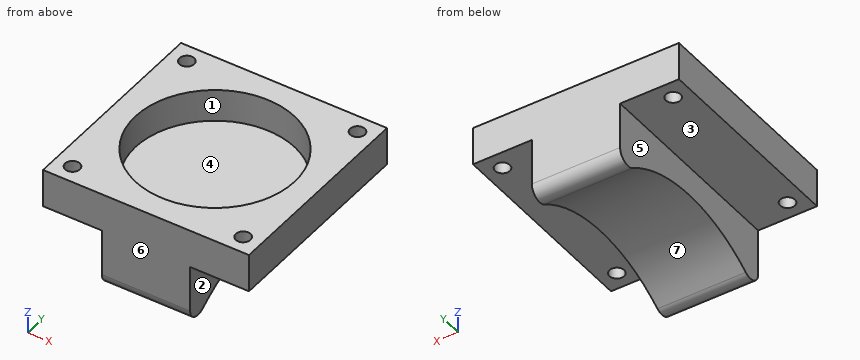
```python
from build123d import *

# Parameters (mm, degrees)
F0_W       = 35
F0_H       = 35
F0_W_2     = 23
F0_H_2     = 23
F1_DEPTH   = 2
F3_DEPTH   = 5.5
F4_DEPTH   = 2.5
F5_DEPTH   = 1
F7_W       = 35
F7_H       = 35
F7_R       = 13.5
F8_DEPTH   = 1
F9_D       = 2.5
F9_DEPTH   = 10
F9_TIP     = 0.7510757738
F9_2_D     = 2.5
F9_2_DEPTH = 10
F9_2_TIP   = 0.7510757738
F10_W      = 7.5
F10_H      = 17.5
F11_DEPTH  = 25
F12_R      = 25
F13_DEPTH  = 25
F14_R      = 2


with BuildPart() as f1:
    # F0 (on Top) → F1 (new body)
    with BuildSketch(Plane.XY):
        with Locations((-9.5, 9.5)):
            Rectangle(F0_W, F0_H)
        with Locations((-9.5, 9.5)):
            Rectangle(F0_W_2, F0_H_2, mode=Mode.SUBTRACT)
        with Locations((-9.5, 9.5)):
            Rectangle(F0_W_2, F0_H_2)
        with BuildLine():
            Line((0, 5.027864045), (0, 0))
            Line((0, 0), (-5.027864045, 0))
            ThreePointArc((-5.027864045, 0), (-9.5, -1), (-13.972135955, 0))
            Line((-13.972135955, 0), (-19, 0))
            Line((-19, 0), (-19, 5.027864045))
            ThreePointArc((-19, 5.027864045), (-20, 9.5), (-19, 13.972135955))
            Line((-19, 13.972135955), (-19, 19))
            Line((-19, 19), (-13.972135955, 19))
            ThreePointArc((-13.972135955, 19), (-9.5, 20), (-5.027864045, 19))
            Line((-5.027864045, 19), (0, 19))
            Line((0, 19), (0, 13.972135955))
            ThreePointArc((0, 13.972135955), (0.746950766, 11.7912878475), (1, 9.5))
            ThreePointArc((1, 9.5), (0.746950766, 7.2087121525), (0, 5.027864045))
        make_face(mode=Mode.SUBTRACT)
        with BuildLine():
            Line((-13.972135955, 0), (-5.027864045, 0))
            ThreePointArc((-5.027864045, 0), (-2.0753787975, 2.0753787975), (0, 5.027864045))
            Line((0, 5.027864045), (0, 13.972135955))
            ThreePointArc((0, 13.972135955), (-2.0753787975, 16.9246212025), (-5.027864045, 19))
            Line((-5.027864045, 19), (-13.972135955, 19))
            ThreePointArc((-13.972135955, 19), (-16.9246212025, 16.9246212025), (-19, 13.972135955))
            Line((-19, 13.972135955), (-19, 5.027864045))
            ThreePointArc((-19, 5.027864045), (-16.9246212025, 2.0753787975), (-13.972135955, 0))
        make_face()
        with BuildLine():
            Line((-19, 19), (-19, 13.972135955))
            ThreePointArc((-19, 13.972135955), (-16.9246212025, 16.9246212025), (-13.972135955, 19))
            Line((-13.972135955, 19), (-19, 19))
        make_face()
        with BuildLine():
            ThreePointArc((-5.027864045, 19), (-2.0753787975, 16.9246212025), (0, 13.972135955))
            Line((0, 13.972135955), (0, 19))
            Line((0, 19), (-5.027864045, 19))
        make_face()
        with BuildLine():
            Line((-5.027864045, 0), (0, 0))
            Line((0, 0), (0, 5.027864045))
            ThreePointArc((0, 5.027864045), (-2.0753787975, 2.0753787975), (-5.027864045, 0))
        make_face()
        with BuildLine():
            Line((-19, 0), (-13.972135955, 0))
            ThreePointArc((-13.972135955, 0), (-16.9246212025, 2.0753787975), (-19, 5.027864045))
            Line((-19, 5.027864045), (-19, 0))
        make_face()
        with BuildLine():
            Line((0, 13.972135955), (0, 5.027864045))
            ThreePointArc((0, 5.027864045), (0.746950766, 7.2087121525), (1, 9.5))
            ThreePointArc((1, 9.5), (0.746950766, 11.7912878475), (0, 13.972135955))
        make_face()
        with BuildLine():
            ThreePointArc((-13.972135955, 0), (-9.5, -1), (-5.027864045, 0))
            Line((-5.027864045, 0), (-13.972135955, 0))
        make_face()
        with BuildLine():
            ThreePointArc((-19, 13.972135955), (-20, 9.5), (-19, 5.027864045))
            Line((-19, 5.027864045), (-19, 13.972135955))
        make_face()
        with BuildLine():
            Line((-13.972135955, 19), (-5.027864045, 19))
            ThreePointArc((-5.027864045, 19), (-9.5, 20), (-13.972135955, 19))
        make_face()
    extrude(amount=-F1_DEPTH)

    # F0 (on Top) → F4 (join)
    with BuildSketch(Plane.XY):
        with Locations((-9.5, 9.5)):
            Rectangle(F0_W_2, F0_H_2)
        with BuildLine():
            Line((0, 5.027864045), (0, 0))
            Line((0, 0), (-5.027864045, 0))
            ThreePointArc((-5.027864045, 0), (-9.5, -1), (-13.972135955, 0))
            Line((-13.972135955, 0), (-19, 0))
            Line((-19, 0), (-19, 5.027864045))
            ThreePointArc((-19, 5.027864045), (-20, 9.5), (-19, 13.972135955))
            Line((-19, 13.972135955), (-19, 19))
            Line((-19, 19), (-13.972135955, 19))
            ThreePointArc((-13.972135955, 19), (-9.5, 20), (-5.027864045, 19))
            Line((-5.027864045, 19), (0, 19))
            Line((0, 19), (0, 13.972135955))
            ThreePointArc((0, 13.972135955), (0.746950766, 11.7912878475), (1, 9.5))
            ThreePointArc((1, 9.5), (0.746950766, 7.2087121525), (0, 5.027864045))
        make_face(mode=Mode.SUBTRACT)
        with BuildLine():
            ThreePointArc((-19, 13.972135955), (-20, 9.5), (-19, 5.027864045))
            Line((-19, 5.027864045), (-19, 13.972135955))
        make_face()
        with BuildLine():
            Line((-13.972135955, 19), (-5.027864045, 19))
            ThreePointArc((-5.027864045, 19), (-9.5, 20), (-13.972135955, 19))
        make_face()
        with BuildLine():
            Line((0, 13.972135955), (0, 5.027864045))
            ThreePointArc((0, 5.027864045), (0.746950766, 7.2087121525), (1, 9.5))
            ThreePointArc((1, 9.5), (0.746950766, 11.7912878475), (0, 13.972135955))
        make_face()
        with BuildLine():
            ThreePointArc((-13.972135955, 0), (-9.5, -1), (-5.027864045, 0))
            Line((-5.027864045, 0), (-13.972135955, 0))
        make_face()
    extrude(amount=F4_DEPTH)


with BuildPart() as f3:
    # F2 (on face) → F3 (new body)
    with BuildSketch(Plane(origin=(0, 0, -2), x_dir=(1, 0, 0), z_dir=(0, 0, -1))):
        with BuildLine():
            Line((-27, -9.5), (-27, -27))
            Line((-27, -27), (8, -27))
            Line((8, -27), (8, -9.5))
            Line((8, -9.5), (4, -9.5))
            ThreePointArc((4, -9.5), (-9.5, -23), (-23, -9.5))
            Line((-23, -9.5), (-27, -9.5))
        make_face()
        with BuildLine():
            Line((-27, 8), (-27, -9.5))
            Line((-27, -9.5), (-23, -9.5))
            ThreePointArc((-23, -9.5), (-9.5, 4), (4, -9.5))
            Line((4, -9.5), (8, -9.5))
            Line((8, -9.5), (8, 8))
            Line((8, 8), (-27, 8))
        make_face()
    extrude(amount=F3_DEPTH)


with BuildPart() as f5:
    # F5 (new): a face of the model
    f5_faces = [f3.part.faces().sort_by_distance(p)[0] for p in [
        (-9.5, 26.5050252532, -7.5),
    ]]
    extrude(f5_faces, amount=F5_DEPTH)


with BuildPart() as f5b:
    # F5#2 (new): a face of the model
    f5_2_faces = [f1.part.faces().sort_by_distance(p)[0] for p in [
        (-9.5, 9.5, -2),
    ]]
    extrude(f5_2_faces, amount=F5_DEPTH)


with BuildPart() as f3_1:
    add(f3.part)

    # F7 (on face) → F8 (join)
    with BuildSketch(Plane(origin=(0, 0, -7.5), x_dir=(1, 0, 0), z_dir=(0, 0, -1))):
        with Locations((-9.5, -9.5)):
            Rectangle(F7_W, F7_H)
        with Locations((-9.5, -9.5)):
            Circle(F7_R, mode=Mode.SUBTRACT)
        with Locations((-9.5, -9.5)):
            Circle(F7_R)
    extrude(amount=F8_DEPTH)

    # F9#2
    with Locations(Plane.XY):
        with Locations((-24, -5), (-24, 24), (5, 24), (5, -5)):
            Hole(F9_2_D / 2, depth=F9_2_DEPTH)
            with Locations((0, 0, -(F9_2_DEPTH + F9_2_TIP / 2))):  # 118° drill point
                Cone(0, F9_2_D / 2, F9_2_TIP, mode=Mode.SUBTRACT)

    # F10 (on face) → F11 (join)
    with BuildSketch(Plane(origin=(0, 0, -8.5), x_dir=(1, 0, 0), z_dir=(0, 0, -1))):
        with Locations((-13.25, -0.75)):
            Rectangle(F10_W, F10_H)
        with Locations((-13.25, -18.25)):
            Rectangle(F10_W, F10_H)
        Polygon((-2, 8), (-9.5, 8), (-9.5, -9.5), (-9.5, -27), (-2, -27), (-2, -9.5), align=None)
    extrude(amount=F11_DEPTH)

    # F12 (on face) → F13 (cut)
    with BuildSketch(Plane(origin=(-17, 0, 0), x_dir=(0, -1, 0), z_dir=(-1, 0, 0))):
        with Locations((-9.5, -38.5)):
            Circle(F12_R)
    extrude(amount=-F13_DEPTH, mode=Mode.SUBTRACT)

    # F14
    f14_edges = [f3_1.edges().sort_by_distance(p)[0] for p in [
        (-9.5, -8, -20.646429),
        (-9.5, 27, -20.646429),
    ]]
    fillet(f14_edges, radius=F14_R)


with BuildPart() as f1_1:
    add(f1.part)

    # F9
    with Locations(Plane.XY):
        with Locations((-24, -5), (-24, 24), (5, 24), (5, -5)):
            Hole(F9_D / 2, depth=F9_DEPTH)
            with Locations((0, 0, -(F9_DEPTH + F9_TIP / 2))):  # 118° drill point
                Cone(0, F9_D / 2, F9_TIP, mode=Mode.SUBTRACT)


solid = f3_1.part
```
Source: CAD feature listing. Evaluate the final solid. Frame: model axes, mm. Face numbers are marked on the shaded views. A direction names the side the tool comes from. Give positions to 0.01 mm unless a question says otherwise; leave off trailing zeros. Write each loop counter-clockwise with the first axis right and the second up, starting at its lowest first coordinate (ties: lowest second). Pieces come first, ordered by that corner, then holes.
1. Material intervals for line 1 along Y through (x, z) = (-24, -6.25); line 2 along X through (y, z) = (9.5, -4.5); line 3 along Y through (x, z) = (-9, -6.25), sorted ascending.
2. Section query A-A (x = -24). Return the cut outline in (y, z).
3. Section query C-C (y = 9.5). Return the cut outline in (x, z), then the cut area to 3 significant figures.
4. Pull-direction query (Y, two-part tool) for the marked faces 4, 5, 6 and 7; classes: +Y half, -Y half, draft (parallel to the pull), parting line (faces both ways), or undercut.
5. Section query B-B (z = -6). Return the cut outline in (x, y), then the cut area to 3 significant figures.
6. Section query D-D (x = -16.5). Return the cut outline in (y, z).
7. First-contact query: pin 1 (8 mm diameter, centred on x = -20.5, y = 11.5, fed in from -Z); pin 2 (1.5 mm diameter, centred on x = -17, y = 1.5, fed in from -Z); pin 3 (11 mm diameter, centred on x = 4.5, y = 15, fed in from -Z). Flat tips, straight axial feed; report the tip coordinate or a pass-through.
8. Access query for the marked faces 1, 2 and 3. Directions: +Z, -Z, +X, -X, +Y, -Y. A direction counts if a zero-diameter tool reaches every point of the face in a straight line with its end or side. Return the directions, or none.
Output values:
1. line 1: y = -8 to -6.25, -3.75 to 22.75, 25.25 to 27
1. line 2: x = -27 to -23, 4 to 8
1. line 3: y = -8 to -3.99, 22.99 to 27
2. outline: (-8, -8.5) - (-6.25, -8.5) - (-6.25, -2) - (-8, -2) - close; (-3.75, -8.5) - (22.75, -8.5) - (22.75, -2) - (-3.75, -2) - close; (25.25, -8.5) - (27, -8.5) - (27, -2) - (25.25, -2) - close
3. outline: (-27, -8.5) - (-17, -8.5) - (-17, -13.5) - (-2, -13.5) - (-2, -8.5) - (8, -8.5) - (8, -2) - (4, -2) - (4, -7.5) - (-23, -7.5) - (-23, -2) - (-27, -2) - close
3. area: 154 mm2
4. face 4: undercut
4. face 5: draft
4. face 6: -Y half
4. face 7: undercut
5. outline: (-27, -8) - (8, -8) - (8, 27) - (-27, 27) - close; hole circle Ø2.5 at (-24, -5); hole circle Ø2.5 at (-24, 24); hole circle Ø27 at (-9.5, 9.5); hole circle Ø2.5 at (5, -5); hole circle Ø2.5 at (5, 24)
5. area: 633 mm2
6. outline: (-8, -16.39) arc R2 ccw to (-4.85, -18.03) arc R25 cw to (23.85, -18.03) arc R2 ccw to (27, -16.39) - (27, -2) - (21.04, -2) - (21.04, -7.5) - (-2.04, -7.5) - (-2.04, -2) - (-8, -2) - close
7. pin 1: stops at z = -13.81
7. pin 2: stops at z = -15.08
7. pin 3: stops at z = -8.5
8. face 1: +Z
8. face 2: -Z, +X, +Y, -Y
8. face 3: -Z, -X, +Y, -Y
